from build123d import *

# Parameters (mm, degrees)
CYLINDER001_R     = 3
CYLINDER001_DEPTH = 10
SKETCH001_R       = 3.4
PAD_DEPTH         = 3
ARRAY001_COUNT    = 8
BOX001_W          = 56
BOX001_H          = 56
BOX001_DEPTH      = 5
SKETCH002_R       = 2
POCKET001_DEPTH   = 2
SKETCH004_R       = 1
POCKET002_DEPTH   = 5.001
SKETCH005_R       = 1
POCKET003_DEPTH   = 5.001


with BuildPart() as array001:
    # Cylinder001 → Cylinder001 (new body)
    with BuildSketch(Plane(origin=(-23.5, 1, 0), x_dir=(1, 0, 0), z_dir=(0, 0, 1))):
        Circle(CYLINDER001_R)
    extrude(amount=CYLINDER001_DEPTH)

    # Sketch001 → Pad (new body, symmetric)
    with BuildSketch(Plane(origin=(-23.5, 1, 0), x_dir=(1, 0, 0), z_dir=(0, 0, -1))):
        Circle(SKETCH001_R)
    extrude(amount=PAD_DEPTH, both=True)

    # Array001: Array001 ×8 about axis
    array001_axis = Axis((0, 0, 0), (0, 0, 1))


with BuildPart() as array001_1:
    add(array001.part)
    for i in range(1, ARRAY001_COUNT):
        add(array001.part.rotate(array001_axis, i * 360 / ARRAY001_COUNT))


with BuildPart() as pocket003:
    # Box001 → Box001 (new body)
    with BuildSketch(Plane(origin=(-28, -28, -5), x_dir=(1, 0, 0), z_dir=(0, 0, 1))):
        with Locations((28, 28)):
            Rectangle(BOX001_W, BOX001_H)
    extrude(amount=BOX001_DEPTH)

    # Fusion: union Array001
    add(array001_1.part)

    # Sketch002 → Pocket001 (cut)
    with BuildSketch(Plane.XY):
        with Locations((-24, 24)):
            Circle(SKETCH002_R)
        with Locations((24, 24)):
            Circle(SKETCH002_R)
        with Locations((24, -24)):
            Circle(SKETCH002_R)
        with Locations((-24, -24)):
            Circle(SKETCH002_R)
    extrude(amount=-POCKET001_DEPTH, mode=Mode.SUBTRACT)

    # Sketch004 → Pocket002 (cut, through all)
    with BuildSketch(Plane.XY):
        with Locations((-24, 24)):
            Circle(SKETCH004_R)
        with Locations((24, 24)):
            Circle(SKETCH004_R)
        with Locations((-24, -24)):
            Circle(SKETCH004_R)
    extrude(amount=-POCKET002_DEPTH, mode=Mode.SUBTRACT)

    # Sketch005 → Pocket003 (cut, through all)
    with BuildSketch(Plane.XY):
        with Locations((24, -24)):
            Circle(SKETCH005_R)
    extrude(amount=-POCKET003_DEPTH, mode=Mode.SUBTRACT)


solid = pocket003.part
Build history of the part. All positions in model axes, mm. A direction names the side the tool comes from. Round coordinates to 2 decimals unless told otherwise and drop trailing zeros. Write each loop counter-clockwise with the first axis right and the second up, starting at its lowest first coordinate (ties: lowest second). Pieces come first, ordered by that corner, then holes. Notation, with made-up numbers: M -34.75,-19 L -29.75,-19 A34 ccw -29.75,15 Z; hole C 3.25,-34.5 d4. An arc over 180 degrees is marked long. Answer as a JSON object with one key per item and string values. Group by question number.
(1) Mould opens along X. For faces 3 (the flat face through (-16, 17, 10)), 4 (the cylindrical face through (0.8, -25.9, 6.5)), 5 (the cylindrical face through (22, -24, -1)) say: pulls with the +X half, pulls with the -X half, needs draft (parallel to the pull), parting line crosses it, or undercut.
(2) Flat gauge pins, fed straight in: pin 1 (3 mm diameter, centred on x = 23, y = -24, fed in from +Z); pin 2 (2 mm diameter, centred on y = -18.5, z = 0.5, fed in from +X); pin 3 (3.5 mm diameter, centred on x = 24, y = -24, fed in from +Z); pin 4 (1.8 mm diameter, centred on x = -24, y = 24, fed in from +Z). Where does each tip first touch, or does it go through?
(3) Cut at C-C (y = 24). Give the cut face in (x, z).
(4) Drill centre lines: L1, parallel to Y at x = -24, z = -4.2; L2, parallel to Y at x = 24, z = -0.75; L3, parallel to Y at x = -17.5, z = 2. Where is each one in solid material? Low to high.
(5) Cut at B-B (x = 24). Give the cut face in (y, z).
(6) Cut at D-D (z = 5.25). Give the cut face in (x, y).
(7) Which spindle directions (+Z, -Z, +X, -X, +Y, -Y) get a long thin tool onto all of the face, cutting with end or side? Do faces 1 (the flat face through (25, -25, -2)), 2 (the cylindrical face through (-24, 23, -3)). Say none if no direction does.
(8) Cut at A-A (z = -1.25). Give the cut face in (x, y).
Responses:
{
 "1": {"face 3": "needs draft", "face 4": "parting line crosses it", "face 5": "undercut"},
 "2": {"pin 1": "stops at z = 0", "pin 2": "stops at x = 28", "pin 3": "stops at z = -2", "pin 4": "passes through"},
 "3": {"outline": "M -28,-5 L -25,-5 L -25,-2 L -26,-2 L -26,0 L -28,0 Z; M -23,-5 L 23,-5 L 23,-2 L 22,-2 L 22,0 L 4.36,0 L 4.36,3 L 3.96,3 L 3.96,10 L -1.96,10 L -1.96,3 L -2.36,3 L -2.36,0 L -22,0 L -22,-2 L -23,-2 Z; M 25,-5 L 28,-5 L 28,0 L 26,0 L 26,-2 L 25,-2 Z"},
 "4": {"L1": "y = -28 to -25, -23 to 23, 25 to 28", "L2": "y = -28 to -26, -22 to 22, 26 to 28", "L3": "y = -19.31 to -12.51, 14.32 to 20.33"},
 "5": {"outline": "M -28,-5 L -25,-5 L -25,-2 L -26,-2 L -26,0 L -28,0 Z; M -23,-5 L 23,-5 L 23,-2 L 22,-2 L 22,0 L 2.36,0 L 2.36,3 L 1.96,3 L 1.96,10 L -3.96,10 L -3.96,3 L -4.36,3 L -4.36,0 L -22,0 L -22,-2 L -23,-2 Z; M 25,-5 L 28,-5 L 28,0 L 26,0 L 26,-2 L 25,-2 Z"},
 "6": {"outline": "C -23.5,1 d6; C -17.32,-15.91 d6; C -15.91,17.32 d6; C -1,-23.5 d6; C 1,23.5 d6; C 15.91,-17.32 d6; C 17.32,15.91 d6; C 23.5,-1 d6"},
 "7": {"face 1": "+Z", "face 2": "+Z, -Z"},
 "8": {"outline": "M -28,-28 L 28,-28 L 28,28 L -28,28 Z; hole C -24,-24 d4; hole C -24,24 d4; hole C 24,-24 d4; hole C 24,24 d4"}
}
